from build123d import *

# Parameters (mm, degrees)
BOSS_EXTRUDE1_DEPTH   = 5
CHAMFER1_SIZE         = 6
CUT_EXTRUDE2_DEPTH    = 6
CHAMFER3_SIZE         = 1
CHAMFER3_SIZE2        = 0.577350269
CHAMFER3_PART_2_SIZE  = 1
CHAMFER3_PART_2_SIZE2 = 0.577350269
CHAMFER3_PART_3_SIZE  = 1
CHAMFER3_PART_3_SIZE2 = 0.577350269
CHAMFER4_SIZE         = 1
CHAMFER4_SIZE2        = 0.577350269
CHAMFER4_PART_2_SIZE  = 1
CHAMFER4_PART_2_SIZE2 = 0.577350269
CHAMFER4_PART_3_SIZE  = 1
CHAMFER4_PART_3_SIZE2 = 0.577350269
FILLET1_R             = 0.8


with BuildPart() as part:
    # Sketch1 → Boss-Extrude1 (new body)
    with BuildSketch(Plane.XY):
        with BuildLine():
            Line((-250.8, 3.6), (-241, 3.6))
            Line((-241, 3.6), (-241, 7.6))
            Line((-241, 7.6), (-233.98, 7.6))
            Line((-233.98, 7.6), (-233.98, 2.6))
            Line((-233.98, 2.6), (-236, 2.6))
            Line((-236, 2.6), (-236, 2.1))
            Line((-236, 2.1), (-235.25, 2.1))
            Line((-235.25, 2.1), (-235.25, -0.4))
            Line((-235.25, -0.4), (-233.98, -0.4))
            Line((-233.98, -0.4), (-233.98, -2.4))
            Line((-233.98, -2.4), (-231.02, -2.4))
            Line((-231.02, -2.4), (-231.02, -0.4))
            Line((-231.02, -0.4), (-229.75, -0.4))
            Line((-229.75, -0.4), (-229.75, 2.1))
            Line((-229.75, 2.1), (-229, 2.1))
            Line((-229, 2.1), (-229, 2.6))
            Line((-229, 2.6), (-231.02, 2.6))
            Line((-231.02, 2.6), (-231.02, 7.6))
            Line((-231.02, 7.6), (-198, 7.6))
            Line((-198, 7.6), (-198, 3.4))
            Line((-198, 3.4), (-183.5, 3.4))
            Line((-183.5, 3.4), (-183.5, 7.6))
            Line((-183.5, 7.6), (-169.5, 7.6))
            Line((-169.5, 7.6), (-169.5, 12.6))
            Line((-169.5, 12.6), (-160.5, 12.6))
            Line((-160.5, 12.6), (-160.5, 7.6))
            Line((-160.5, 7.6), (-139.25, 7.6))
            Line((-139.25, 7.6), (-139.25, 3.4))
            Line((-139.25, 3.4), (-124.75, 3.4))
            Line((-124.75, 3.4), (-124.75, 7.6))
            Line((-124.75, 7.6), (-80.5, 7.6))
            Line((-80.5, 7.6), (-80.5, 3.4))
            Line((-80.5, 3.4), (-66, 3.4))
            Line((-66, 3.4), (-66, 7.6))
            Line((-66, 7.6), (-13.75, 7.6))
            Line((-13.75, 7.6), (-13.75, 12.6))
            Line((-13.75, 12.6), (-4.25, 12.6))
            Line((-4.25, 12.6), (-4.25, 7.6))
            Line((-4.25, 7.6), (20, 7.6))
            Line((20, 7.6), (20, 0))
            Line((20, 0), (0, 0))
            Line((0, 0), (0, -11.4))
            Line((0, -11.4), (-221.799463771, -11.4))
            ThreePointArc((-221.799463771, -11.4), (-223.557706142, -11.555784248), (-225.261167219, -12.018283247))
            ThreePointArc((-225.261167219, -12.018283247), (-232.5, -13.3111869), (-239.738832781, -12.018283247))
            ThreePointArc((-239.738832781, -12.018283247), (-241.442293858, -11.555784248), (-243.200536229, -11.4))
            Line((-243.200536229, -11.4), (-287.270831989, -11.4))
            ThreePointArc((-287.270831989, -11.4), (-289.270831989, -13.4), (-287.270831989, -15.4))
            Line((-287.270831989, -15.4), (-282, -15.4))
            Line((-282, -15.4), (-282, -18.281197846))
            Line((-282, -18.281197846), (-283, -20.013248654))
            Line((-283, -20.013248654), (-286, -18.281197846))
            Line((-286, -18.281197846), (-290, -20.590598923))
            Line((-290, -20.590598923), (-290, -25.209401077))
            Line((-290, -25.209401077), (-286, -27.518802154))
            Line((-286, -27.518802154), (-283, -25.786751346))
            Line((-283, -25.786751346), (-282, -27.518802154))
            Line((-282, -27.518802154), (-282, -30.9))
            Line((-282, -30.9), (-297.5, -30.9))
            Line((-297.5, -30.9), (-297.5, -8.4))
            Line((-297.5, -8.4), (-292.5, -8.4))
            Line((-292.5, -8.4), (-292.5, 1.6))
            Line((-292.5, 1.6), (-298.5, 7.6))
            Line((-298.5, 7.6), (-299.5, 7.6))
            Line((-299.5, 7.6), (-299.5, 12.6))
            Line((-299.5, 12.6), (-290, 12.6))
            Line((-290, 12.6), (-290, 7.6))
            Line((-290, 7.6), (-259.093151184, 7.6))
            Line((-259.093151184, 7.6), (-259.093151184, 5.6))
            Line((-259.093151184, 5.6), (-255.2, 5.6))
            Line((-255.2, 5.6), (-255.2, 3.1))
            Line((-255.2, 3.1), (-250.8, 3.1))
            Line((-250.8, 3.1), (-250.8, 3.6))
        make_face()
    extrude(amount=BOSS_EXTRUDE1_DEPTH)

    # Chamfer1
    chamfer1_edges = [part.edges().sort_by_distance(p)[0] for p in [
        (0, -11.4, 2.5),
    ]]
    chamfer(chamfer1_edges, length=CHAMFER1_SIZE)

    # Sketch3 → Cut-Extrude2 (cut, through all)
    with BuildSketch(Plane.XY.offset(5)):
        Polygon((-289.270831989, -13.4), (-289.270831989, -15.4), (-297.5, -15.4), (-297.5, -30.9), (-282, -30.9), (-282, -13.4), align=None)
    extrude(amount=-CUT_EXTRUDE2_DEPTH, mode=Mode.SUBTRACT)

    # Chamfer3
    chamfer3_edges = [part.edges().sort_by_distance(p)[0] for p in [
        (-290, 12.6, 2.5),
    ]]
    chamfer3_side = [part.faces().sort_by_distance(p)[0] for p in [
        (-290, 10.1, 2.5),
    ]]
    chamfer(chamfer3_edges, length=CHAMFER3_SIZE, length2=CHAMFER3_SIZE2, reference=chamfer3_side[0])

    # Chamfer3 part 2
    chamfer3_part_2_edges = [part.edges().sort_by_distance(p)[0] for p in [
        (-160.5, 12.6, 2.5),
    ]]
    chamfer3_part_2_side = [part.faces().sort_by_distance(p)[0] for p in [
        (-160.5, 10.1, 2.5),
    ]]
    chamfer(chamfer3_part_2_edges, length=CHAMFER3_PART_2_SIZE, length2=CHAMFER3_PART_2_SIZE2, reference=chamfer3_part_2_side[0])

    # Chamfer3 part 3
    chamfer3_part_3_edges = [part.edges().sort_by_distance(p)[0] for p in [
        (-4.25, 12.6, 2.5),
    ]]
    chamfer3_part_3_side = [part.faces().sort_by_distance(p)[0] for p in [
        (-4.25, 10.1, 2.5),
    ]]
    chamfer(chamfer3_part_3_edges, length=CHAMFER3_PART_3_SIZE, length2=CHAMFER3_PART_3_SIZE2, reference=chamfer3_part_3_side[0])

    # Chamfer4
    chamfer4_edges = [part.edges().sort_by_distance(p)[0] for p in [
        (-299.5, 12.6, 2.5),
    ]]
    chamfer4_side = [part.faces().sort_by_distance(p)[0] for p in [
        (-299.5, 10.1, 2.5),
    ]]
    chamfer(chamfer4_edges, length=CHAMFER4_SIZE, length2=CHAMFER4_SIZE2, reference=chamfer4_side[0])

    # Chamfer4 part 2
    chamfer4_part_2_edges = [part.edges().sort_by_distance(p)[0] for p in [
        (-169.5, 12.6, 2.5),
    ]]
    chamfer4_part_2_side = [part.faces().sort_by_distance(p)[0] for p in [
        (-169.5, 10.1, 2.5),
    ]]
    chamfer(chamfer4_part_2_edges, length=CHAMFER4_PART_2_SIZE, length2=CHAMFER4_PART_2_SIZE2, reference=chamfer4_part_2_side[0])

    # Chamfer4 part 3
    chamfer4_part_3_edges = [part.edges().sort_by_distance(p)[0] for p in [
        (-13.75, 12.6, 2.5),
    ]]
    chamfer4_part_3_side = [part.faces().sort_by_distance(p)[0] for p in [
        (-13.75, 10.1, 2.5),
    ]]
    chamfer(chamfer4_part_3_edges, length=CHAMFER4_PART_3_SIZE, length2=CHAMFER4_PART_3_SIZE2, reference=chamfer4_part_3_side[0])

    # Fillet1
    fillet1_edges = [part.edges().sort_by_distance(p)[0] for p in [
        (-198, 3.4, 2.5),
        (-183.5, 3.4, 2.5),
        (-139.25, 3.4, 2.5),
        (-124.75, 3.4, 2.5),
        (-80.5, 3.4, 2.5),
        (-66, 3.4, 2.5),
    ]]
    fillet(fillet1_edges, radius=FILLET1_R)


solid = part.part
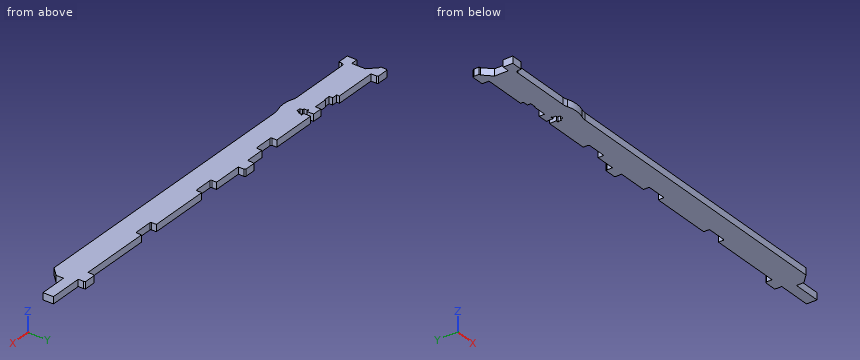
Source: CAD feature listing. Evaluate the final solid. Frame: model axes, mm. Round coordinates to 2 decimals unless told otherwise and drop trailing zeros. Loops run counter-clockwise (first coordinate to the right, second up) from the corner with the lowest first, then second, coordinate; pieces in that order, holes last. Notation, with made-up numbers: (75.5, -6.5) -> (131.5, -6.5) arc R12 ccw to (131.5, 15.5) -> close; hole circle Ø5 at (18, -6.75). An arc over 180 degrees is marked (long way). Answer as a JSON object with one key per item and string values. Group by question number.
Q1. Ray query, line 1 (X direction, y = 9, z = 4.1); line 2 (X direction, y = 7, z = 1.2); line 3 (X direction, y = -2, z = 3.3). Return the intervals inside material, ascending. Write a range as from..to.
Q2. Contact query for flat-ended pins moving along their axis: P1, Ø3, axis at x = -204.5, z = 1.5, coming from the -Y side; P2, Ø2.5, axis at x = -189.5, z = 1.5, coming from the +Y side; P3, Ø1.5, axis at x = -268.5, z = 1.5, coming from the +Y side. Output: stop coordinate, or through.
Q3. Section query A-A (x = -211). Output: boundary loops of the cut face in (y, z), plus the area to 3 significant figures.
Completed:
{
 "1": {"line 1": "-299.5..-290, -169.5..-160.5, -13.75..-4.25", "line 2": "-297.9..-259.09, -241..-233.98, -231.02..-198, -183.5..-139.25, -124.75..-80.5, -66..20", "line 3": "-292.5..-233.98, -231.02..0"},
 "2": {"P1": "y = -11.4", "P2": "y = 3.4", "P3": "y = 7.6"},
 "3": {"outline": "(-11.4, 0) -> (7.6, 0) -> (7.6, 5) -> (-11.4, 5) -> close", "area": "95.0 mm²"}
}
